Here's the drawing with two shaded views (mm, measured from the low corner). I have some questions. A direction names the side the tool comes from. Coordinates: 2 decimals unless noted, no trailing zeros. Order: outer loops, then holes, each group sorted by start corner. A loop starts at its lowest first (then second) coordinate and runs counter-clockwise, first axis right, second up. Notation, with made-up numbers: (-11, 18) -> (44, 18) arc R24 cw to (44, 29) -> close; hole circle Ø6 at (-5.75, 1.25). An arc over 180 degrees is marked (long way). Write item = value, one per line.
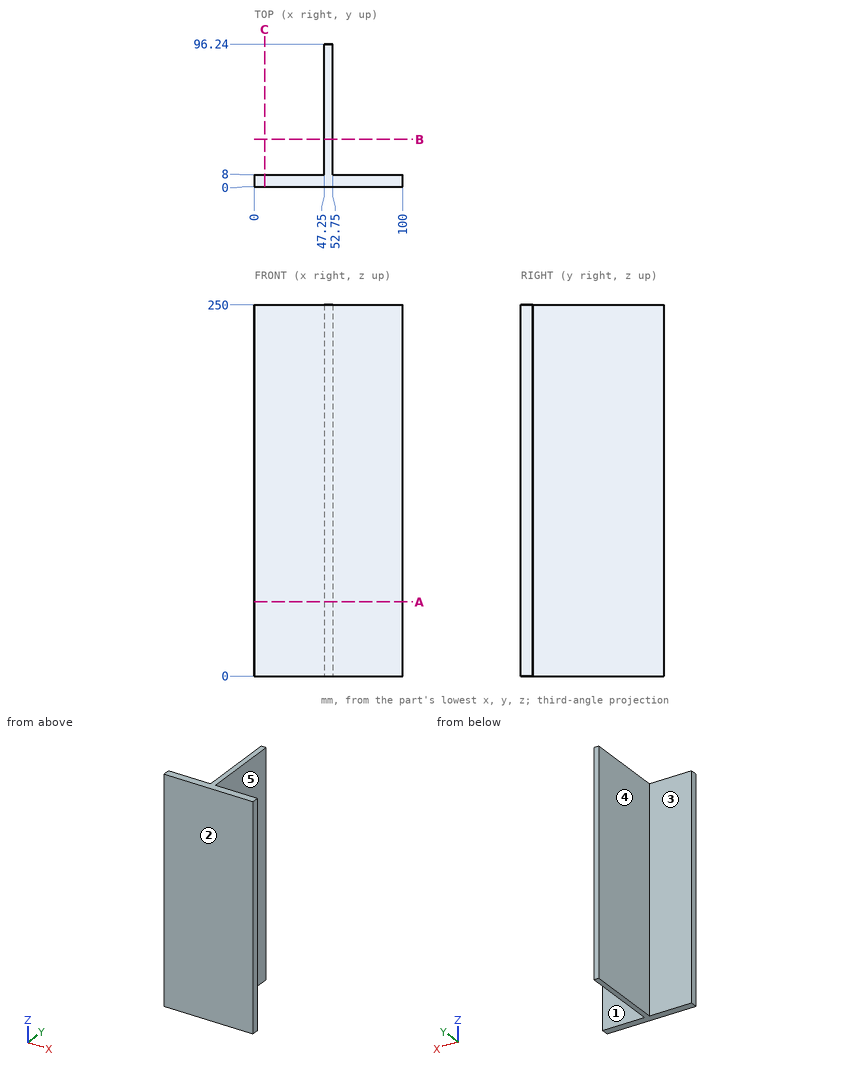
Item 1: If I drill on probe 1 along X at (y, z) = (39, 198); probe 2 along Y at (x, z) = (12, 145.5), over which ranges is the centre line in solid material (lowest first)?
A:
probe_1 = 47.25 to 52.75
probe_2 = 0 to 8
Item 2: I want a section at A-A, the plane z = 50. Please give me the cut outline in (x, y).
A:
outline = (0, 0) -> (100, 0) -> (100, 8) -> (52.75, 8) -> (52.75, 96.24) -> (47.25, 96.24) -> (47.25, 8) -> (0, 8) -> close
Item 3: If we mould it in two halves opening along X, with no side actions, what happens to the marked faces 3, 4 and 5? For each: pulls with the +X half, pulls with the -X half, needs draft (parallel to the pull), parting line crosses it, or undercut.
A:
face_3 = needs draft
face_4 = pulls with the -X half
face_5 = pulls with the +X half
Item 4: I want a section at B-B, the plane y = 32. Please give me the cut outline in (x, z).
A:
outline = (47.25, 0) -> (52.75, 0) -> (52.75, 250) -> (47.25, 250) -> close
Item 5: I'm going to push flat-ended pins straight in: P1, Ø6, axis at x = 29, z = 25.5, coming from the +Y side; P2, Ø3, axis at y = 50, z = 202.5, coming from the +X side. Where does each tip first touch, or does it pass through?
A:
P1 = 8
P2 = 52.75
Item 6: I want a section at C-C, the plane x = 7. Please give me the cut outline in (y, z), plus the area to 3 significant figures.
A:
outline = (0, 0) -> (8, 0) -> (8, 250) -> (0, 250) -> close
area = 2,000 mm2
Item 7: For the marked faces 1 and 2, which set-ups out of +Z, -Z, +X, -X, +Y, -Y let a thin tool reach every point of the face, with its end or its side?
A:
face_1 = +Z, -Z, +X, +Y
face_2 = +Z, -Z, +X, -X, -Y
